Verification items for the finished model (mm, model axes). Round coordinates to 2 decimals unless told otherwise and drop trailing zeros. Order: outer loops, then holes, each group sorted by start corner. A loop starts at its lowest first (then second) coordinate and runs counter-clockwise, first axis right, second up. Notation, with made-up numbers: (-24.75, -20.75) -> (13.25, -20.75) arc R24 ccw to (13.25, 8.25) -> close; hole circle Ø4 at (72, 49.25). An arc over 180 degrees is marked (long way). Return JSON: item names as keys, results as strings. Group by question number.
1) Depth check by flat-ended pin: pin 1 (1 mm diameter, centred on x = -34.5, z = 1.5, fed in from +Y); pin 2 (1 mm diameter, centred on x = 19.5, z = 1, fed in from +Y); pin 3 (1.5 mm diameter, centred on y = -31.5, z = 0.5, fed in from +X). Enter the tip coordinate at first touch or a pass-through.
2) Section check D-D on y = -38. Enter the section's corners in (x, z) (3 decimals), plus the area to 3 significant figures.
3) Section check A-A on x = 0. Enter the section's corners in (y, z) (3 decimals).
4) Scan lines: L1, parallel to Y at x = 5, z = 0.3; L2, parallel to X at y = -24, z = 1.6; L3, parallel to X at y = 26.5, z = 2.85. Record each from-to range of solid material in increasing order.
5) Section check B-B on y = -25. Enter the section's corners in (x, z) (3 decimals).
6) Section check C-C on z = 0.9. State how many separate pieces and enclosed holes the cut face has, plus the area to 3 significant figures.
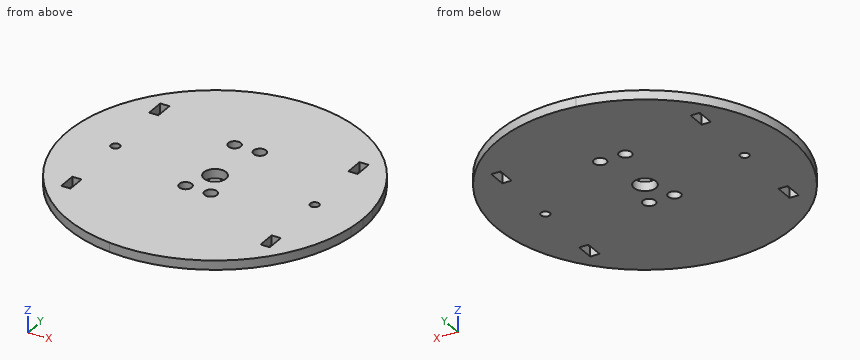
```python
from build123d import *

# Parameters (mm, degrees)
F0_W     = 3.175
F0_H     = 6.35
F0_R     = 1.524
F0_R_2   = 2.159
F0_R_3   = 3.81
F1_DEPTH = 3.175


# Not quite as in the source:
# - a length typed as a fraction of an inch, garbled in the dataset ("3 / 203.2 mm" for 3/8 in), is restored


with BuildPart() as f1:
    # F0 (on Top) → F1 (new body)
    with BuildSketch(Plane.XY):
        with BuildLine():
            ThreePointArc((-50.403125, 6.3375855209), (-50.8, 0), (-50.403125, -6.3375855209))
            ThreePointArc((-50.403125, -6.3375855209), (-35.9210244843, -35.9210244843), (-6.3375855209, -50.403125))
            ThreePointArc((-6.3375855209, -50.403125), (0, -50.8), (6.3375855209, -50.403125))
            ThreePointArc((6.3375855209, -50.403125), (35.9210244843, -35.9210244843), (50.403125, -6.3375855209))
            ThreePointArc((50.403125, -6.3375855209), (50.700684167, -3.175), (50.8, 0))
            ThreePointArc((50.8, 0), (50.700684167, 3.175), (50.403125, 6.3375855209))
            ThreePointArc((50.403125, 6.3375855209), (35.9210244843, 35.9210244843), (6.3375855209, 50.403125))
            ThreePointArc((6.3375855209, 50.403125), (0, 50.8), (-6.3375855209, 50.403125))
            ThreePointArc((-6.3375855209, 50.403125), (-35.9210244843, 35.9210244843), (-50.403125, 6.3375855209))
        make_face()
        with Locations((-34.2304483056, -25.4)):
            Rectangle(F0_W, F0_H, mode=Mode.SUBTRACT)
        with Locations((-34.2304483056, 0)):
            Circle(F0_R, mode=Mode.SUBTRACT)
        with Locations((-4.3434, -9.7282)):
            Circle(F0_R_2, mode=Mode.SUBTRACT)
        Circle(F0_R_3, mode=Mode.SUBTRACT)
        with Locations((34.2304483056, -25.4)):
            Rectangle(F0_W, F0_H, mode=Mode.SUBTRACT)
        with Locations((4.3434, -9.7282)):
            Circle(F0_R_2, mode=Mode.SUBTRACT)
        with Locations((34.2304483056, 0)):
            Circle(F0_R, mode=Mode.SUBTRACT)
        with Locations((-34.2304483056, 25.4)):
            Rectangle(F0_W, F0_H, mode=Mode.SUBTRACT)
        with Locations((-4.3434, 18.6182)):
            Circle(F0_R_2, mode=Mode.SUBTRACT)
        with Locations((4.3434, 18.6182)):
            Circle(F0_R_2, mode=Mode.SUBTRACT)
        with Locations((34.2304483056, 25.4)):
            Rectangle(F0_W, F0_H, mode=Mode.SUBTRACT)
    extrude(amount=F1_DEPTH)


solid = f1.part
```
Check result:
{
 "1": {"pin 1": "y = 37.74", "pin 2": "y = 47.11", "pin 3": "x = 40.44"},
 "2": {"outline": "(-33.714, 0) -> (33.714, 0) -> (33.714, 3.175) -> (-33.714, 3.175) -> close", "area": "214 mm^2"},
 "3": {"outline": "(-50.8, 0) -> (-3.81, 0) -> (-3.81, 3.175) -> (-50.8, 3.175) -> close; (3.81, 0) -> (50.8, 0) -> (50.8, 3.175) -> (3.81, 3.175) -> close"},
 "4": {"L1": "-50.55 to -11.78, -7.67 to 16.56, 20.67 to 50.55", "L2": "-44.77 to -35.82, -32.64 to 32.64, 35.82 to 44.77", "L3": "-43.34 to -35.82, -32.64 to 32.64, 35.82 to 43.34"},
 "5": {"outline": "(-44.223, 0) -> (-35.818, 0) -> (-35.818, 3.175) -> (-44.223, 3.175) -> close; (-32.643, 0) -> (32.643, 0) -> (32.643, 3.175) -> (-32.643, 3.175) -> close; (35.818, 0) -> (44.223, 0) -> (44.223, 3.175) -> (35.818, 3.175) -> close"},
 "6": {"separate pieces": "1", "enclosed holes": "11", "area": "7,910 mm^2"}
}
